Build history of the part. All positions in model axes, mm. A direction names the side the tool comes from. Round coordinates to 2 decimals unless told otherwise and drop trailing zeros. Order: outer loops, then holes, each group sorted by start corner. A loop starts at its lowest first (then second) coordinate and runs counter-clockwise, first axis right, second up. Notation, with made-up numbers: M 0,-25 L 33,-25 A26 cw 33,1 Z; hole C -35.5,87.25 d10. An arc over 180 degrees is marked long. One line per item, written item: value. Start each with the question number.
Item 1: Band-saw the part on B-B, the plane x = 13. Write the cut outline in (y, z), then the cut area to 3 significant figures.
Item 2: Tool access for faces 1 (the cylindrical face through (-1.63, 2.24, 0.04)), 2 (the flat face through (3, 0, 2.5)): list every direction of +Z, -Z, +X, -X, +Y, -Y with a clear straight run to the whole face (end or side of a thin tool).
Item 3: Pin check, flat tips, straight feed: pin 1 (3 mm diameter, centred on x = 10, z = 0, fed in from -Y); pin 2 (2 mm diameter, centred on x = 3, z = 1.5, fed in from +Y); pin 3 (4 mm diameter, centred on x = 0, y = 0, fed in from +Z). Stop position of each tip, or through.
Item 4: Band-saw the part on D-D, the plane y = 3.5. Write the cut outline in (x, z).
Item 5: Probe L1, parallel to Y at x = 0, z = 0.15; L2, parallel to X at y = 0, z = -1; L3, parallel to Y at x = 9.5, z = 0.15. List the from-to ranges inside material, lowest first.
Item 6: Band-saw the part on A-A, the plane x = 0. Write the cut outline in (y, z).
Item 7: Two-plate mould, pull along Y, no slides. Class faces 3 (the cylindrical face through (-2.7, -3.83, -0.04)), 4 (the flat face through (14.886, 0, 0)), 5 (the cylindrical face through (2.5, 0.1, 0)), 6 (the cylindrical face through (9.203, -0.52, -2.343)): +Y half, -Y half, draft (parallel to the pull), parting line (faces both ways), or undercut.
Item 8: Band-saw the part on C-C, the plane z = 0. Write the cut outline in (x, y).
Autodesk Inventor part; units mm, degrees
ref_plane "YZ Plane" through (0, 0, 0) normal (1, 0, 0) x (0, 1, 0)
ref_plane "XZ Plane" through (0, 0, 0) normal (0, 1, 0) x (-1, 0, 0)
ref_plane "XY Plane" through (0, 0, 0) normal (0, 0, 1) x (1, 0, 0)
sketch "Sketch1" plane through (0, 0, 0) normal (0, 0, 1) x (1, 0, 0)
  circle A0 centre (0, 0) radius 5
  circle A1 centre (0, 0) radius 2.5
  line L0 (0, 0) -> (-5, 0) construction
  line L1 (0, 0) -> (-3.213938, 3.830222)
  line L2 (0, 0) -> (-3.213938, -3.830222)
  line L3 (4.386342, 2.4) -> (14.386342, 2.4)
  line L4 (14.386342, 2.4) -> (14.386342, -2.4)
  line L5 (14.386342, -2.4) -> (4.386342, -2.4)
  line L6 (4.386342, -2.4) -> (4.386342, 2.4)
  point P0 (-1.606969, 1.915111)
  point P1 (-1.606969, -1.915111)
  dimension "d0" = 10
  dimension "d1" = 5
  dimension "d2" = 50
  dimension "d3" = 50
  dimension "d4" = 4.8
  dimension "d5" = 10
extrude "Extrusion1" add sketch "Sketch1" along normal mid plane 5 contours A0 L6 | L6 A0 L2 A1 L1
sketch "Sketch2" plane through (0, 0, 0) normal (0, 0, 1) x (1, 0, 0)
  arc A0 (-3.213938, -3.830222) -> (-3.213938, 3.830222) centre (0, 0) ccw construction
  line L0 (4.386342, 2.4) -> (14.886342, 2.4)
  line L1 (14.886342, 2.4) -> (14.886342, -2.4)
  line L2 (14.886342, -2.4) -> (4.386342, -2.4)
  line L3 (4.386342, -2.4) -> (4.386342, 2.4)
  line L4 (4.386342, 0) -> (14.886342, 0)
  dimension "d8" = 4.8
  dimension "d9" = 10.5
revolve "Revolution1" add sketch "Sketch2" angle 360 about axis through (4.386342, 0, 0) along (1, 0, 0) contours L0 L1 L4 L3
chamfer "Chamfer1" distance 1 angle 45 1 edges at (14.8863, -2.4, 0)
fillet "Fillet1" radius 1 4 edges at (-1.607, 1.9151, 0) (-3.2139, 3.8302, 0) (-1.607, -1.9151, 0) (-3.2139, -3.8302, 0)
properties part number "joint_part_black_2"
Output:
1. outline: C 0,0 d4.8
1. area: 18.1 mm²
2. face 1: +Z, -Z
2. face 2: +Z, +X, -X, +Y, -Y
3. pin 1: stops at y = -2.4
3. pin 2: stops at y = 4.58
3. pin 3: passes through
4. outline: M -2.72,-2.5 L 3.57,-2.5 L 3.57,2.5 L -2.72,2.5 Z
5. L1: y = -5 to -2.5, 2.5 to 5
5. L2: x = 2.5 to 14.89
5. L3: y = -2.4 to 2.4
6. outline: M -5,-2.5 L -2.5,-2.5 L -2.5,2.5 L -5,2.5 Z; M 2.5,-2.5 L 5,-2.5 L 5,2.5 L 2.5,2.5 Z
7. face 3: undercut
7. face 4: draft
7. face 5: undercut
7. face 6: parting line
8. outline: M -2.49,-2.97 A1 ccw -2.15,-4.51 A5 ccw 4.39,-2.4 L 13.89,-2.4 L 14.89,-1.4 L 14.89,1.4 L 13.89,2.4 L 4.39,2.4 A5 ccw -2.15,4.51 A1 ccw -2.49,2.97 L -2.16,2.57 A1 ccw -0.99,2.29 A2.5 cw long -0.99,-2.29 A1 ccw -2.16,-2.57 Z
